Autodesk Inventor part; units mm, degrees
ref_plane "YZ Plane" through (0, 0, 0) normal (1, 0, 0) x (0, 1, 0)
ref_plane "XZ Plane" through (0, 0, 0) normal (0, 1, 0) x (-1, 0, 0)
ref_plane "XY Plane" through (0, 0, 0) normal (0, 0, 1) x (1, 0, 0)
sketch "Sketch3" plane through (0, 0, 0) normal (1, 0, 0) x (0, 1, 0)
  line L0 (0, 0) -> (0, 24.2821)
  line L1 (7, 0) -> (7, 5)
  line L2 (7, 5) -> (6.5, 5)
  line L3 (6.5, 5) -> (6.5, 1)
  line L4 (6.5, 1) -> (2.6, 1)
  line L5 (2.6, 1) -> (2.6, 0)
  line L6 (7, 0) -> (2.6, 0)
  dimension "d7" = 5.2
  dimension "d10" = 1
  dimension "d12" = 5
  dimension "d13" = 14
  dimension "d14" = 13
revolve "Revolution1" add sketch "Sketch3" angle 360 about axis through (0, 0, 0) along (0, 0, 1)
fillet "Fillet1" radius 1 1 edges at (0, -7, 0)
equation "\"d10\" = wall_thickness"
equation "\"wall_thickness\" = 1"
properties part number "Electrode Skirt Short" material "Stainless Steel"
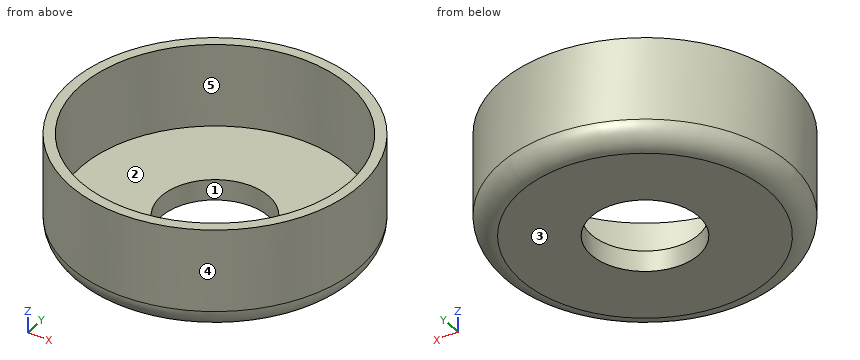
Work out the finished part from the listing and answer in its coordinate system (mm). Face numbers are marked on the shaded views. A direction names the side the tool comes from. Round coordinates to 2 decimals unless told otherwise and drop trailing zeros. Write each loop counter-clockwise with the first axis right and the second up, starting at its lowest first coordinate (ties: lowest second). Pieces come first, ordered by that corner, then holes. Notation, with made-up numbers: (11, -17.75) - (16, -17.75) arc R27 ccw to (16, 7.25) - close; hole circle Ø8 at (4, 55). An arc over 180 degrees is marked (long way). Answer in a Markdown table with one row per item. Add a question column.
1. The mould has two halves that part along Y. Classify the marked faces 3, 4 and 5: +Y half, -Y half, draft (parallel to the pull), parting line (faces both ways), or undercut.
2. Find the intervals of material crossed by line 1 along Y through (x, z) = (0, 3.15); line 2 along Z through (x, y) = (-2.75, 3.5); line 3 along Y through (x, z) = (2, 4.65), in increasing order. Write a range as from..to.
3. A cutting plane is placed at C-C, the plane z = 1.7. Determine the outline of the cut face in (x, y).
4. A cutting plane is placed at A-A, the plane x = 0. Determine the outline of the cut face in (y, z).
5. For the marked faces 1 and 2, determine the directions among +Z, -Z, +X, -X, +Y, -Y from which every point of the face is accessible in a straight line to the end or side of a thin tool.
6. Given pin 1 (1 mm diameter, centred on y = 2, z = 1, fed in from +X); pin 2 (3 mm diameter, centred on y = -3.5, z = 2, fed in from -X); pin 3 (4.5 mm diameter, centred on x = 0, y = 0, fed in from +Z), each flat-ended and moving along its own axis, determine where each tip first touches the part or whether it passes through.
Worked out:
| question | item | result |
|---|---|---|
| 1 | face 3 | draft |
| 1 | face 4 | parting line |
| 1 | face 5 | undercut |
| 2 | line 1 | -7..-6.5, 6.5..7 |
| 2 | line 2 | 0..1 |
| 2 | line 3 | -6.71..-6.18, 6.18..6.71 |
| 3 | outline | circle Ø14 at (0, 0); hole circle Ø13 at (0, 0) |
| 4 | outline | (-7, 1) arc R1 ccw to (-6, 0) - (-2.6, 0) - (-2.6, 1) - (-6.5, 1) - (-6.5, 5) - (-7, 5) - close; (2.6, 0) - (6, 0) arc R1 ccw to (7, 1) - (7, 5) - (6.5, 5) - (6.5, 1) - (2.6, 1) - close |
| 5 | face 1 | +Z, -Z |
| 5 | face 2 | +Z |
| 6 | pin 1 | x = 6.84 |
| 6 | pin 2 | x = -6.71 |
| 6 | pin 3 | through |
